```python
from build123d import *

# Parameters (mm, degrees)
DODANIE_WYCI_GNI_CIE1_DEPTH = 5
DODANIE_WYCI_GNI_CIE2_START = 17
SZKIC3_R                    = 12.625
DODANIE_WYCI_GNI_CIE2_DEPTH = 17
SZKIC4_R                    = 2.5
SZKIC4_R_2                  = 1.55
WYTNIJ_WYCI_GNI_CIE1_DEPTH  = 25
SZKIC5_R                    = 3.75
WYTNIJ_WYCI_GNI_CIE2_DEPTH  = 7.5
DODANIE_WYCI_GNI_CIE3_DEPTH = 15
SZKIC7_R                    = 1.5
WYTNIJ_WYCI_GNI_CIE3_DEPTH  = 14
SZKIC8_R                    = 7.5
WYTNIJ_WYCI_GNI_CIE4_DEPTH  = 14
SZKIC14_R                   = 12.625
SZKIC16_R                   = 10.3
SZKIC18_R                   = 3.75
WYTNIJ_WYCI_GNI_CIE5_DEPTH  = 7.5
SZKIC19_R                   = 0.7
WYTNIJ_WYCI_GNI_CIE6_DEPTH  = 5


with BuildPart() as part:
    # Szkic1 → Dodanie-wyciągnięcie1 (new body)
    with BuildSketch(Plane(origin=(0, 0, 0), x_dir=(1, 0, 0), z_dir=(0, 1, 0))):
        with BuildLine():
            Line((-9, 0), (-9, 55.600537222))
            ThreePointArc((-9, 55.600537222), (7.148204378, 68.984355181), (13.393573335, 48.962206087))
            add(Edge.make_bspline(
                [(0, 21.46), (3.478909601, 36.621824573), (13.393573335, 48.962206087)],
                knots=[0, 0, 0, 1, 1, 1], degree=2))
            Line((0, 21.46), (0, 16.16))
            add(Edge.make_bspline(
                [(0, 16.16), (0.310809708, 10.646673881), (5.027347184, 7.464970214)],
                knots=[0, 0, 0, 1, 1, 1], degree=2))
            ThreePointArc((5.027347184, 7.464970214), (4.228112779, -7.945002349), (-9, 0))
        make_face()
    extrude(amount=DODANIE_WYCI_GNI_CIE1_DEPTH)

    # Szkic3 → Dodanie-wyciągnięcie2 (add)
    with BuildSketch(Plane.XZ.offset(DODANIE_WYCI_GNI_CIE2_START)):
        with Locations(Location((3.56, -56.88, 0), (0, 0, 270))):
            Circle(SZKIC3_R)
    extrude(amount=-DODANIE_WYCI_GNI_CIE2_DEPTH)

    # Szkic4 → Wytnij-wyciągnięcie1 (cut)
    with BuildSketch(Plane.XZ.offset(17)):
        with Locations(Location((3.56, -56.88, 0), (0, 0, 270))):
            Circle(SZKIC4_R)
        with Locations(Location((-3.35, -49.97, 0), (0, 0, 270))):
            Circle(SZKIC4_R_2)
        with Locations(Location((10.47, -49.97, 0), (0, 0, 270))):
            Circle(SZKIC4_R_2)
        with Locations(Location((-3.35, -63.79, 0), (0, 0, 270))):
            Circle(SZKIC4_R_2)
        with Locations(Location((10.47, -63.79, 0), (0, 0, 270))):
            Circle(SZKIC4_R_2)
    extrude(amount=-WYTNIJ_WYCI_GNI_CIE1_DEPTH, mode=Mode.SUBTRACT)

    # Szkic5 → Wytnij-wyciągnięcie2 (cut)
    with BuildSketch(Plane.XZ.offset(17)):
        with Locations(Location((3.56, -56.88, 0), (0, 0, 270))):
            Circle(SZKIC5_R)
    extrude(amount=-WYTNIJ_WYCI_GNI_CIE2_DEPTH, mode=Mode.SUBTRACT)

    # Szkic6 → Dodanie-wyciągnięcie3 (add)
    with BuildSketch(Plane(origin=(0, 5, 0), x_dir=(1, 0, 0), z_dir=(0, 1, 0))):
        with BuildLine():
            Line((-9, 55.600537222), (-9, 62.310537222))
            Line((-9, 62.310537222), (-4.379377966, 68.310537222))
            Line((-4.379377966, 68.310537222), (1.560622034, 69.345677388))
            add(Edge.make_bspline(
                [(1.560622034, 69.345677388), (-7.284103586, 65.531370102), (-9, 55.600537222)],
                knots=[0, 0, 0, 1, 1, 1], degree=2))
        make_face()
    extrude(amount=-DODANIE_WYCI_GNI_CIE3_DEPTH)

    # Szkic7 → Wytnij-wyciągnięcie3 (cut)
    with BuildSketch(Plane(origin=(-35.771148282, 0, -27.547492656), x_dir=(-0.6101451639012687, 0, 0.7922896433551899), z_dir=(-0.7922896433551899, 0, -0.6101451639012687))):
        with Locations((-47.663180862, 2)):
            Circle(SZKIC7_R)
        with Locations((-47.663180862, -7)):
            Circle(SZKIC7_R)
    extrude(amount=-WYTNIJ_WYCI_GNI_CIE3_DEPTH, mode=Mode.SUBTRACT)

    # Szkic8 → Wytnij-wyciągnięcie4 (cut)
    with BuildSketch(Plane(origin=(0, 5, 0), x_dir=(1, 0, 0), z_dir=(0, 1, 0))):
        with Locations(Location((0, 0, 0), (0, 0, 270))):
            Circle(SZKIC8_R)
    extrude(amount=-WYTNIJ_WYCI_GNI_CIE4_DEPTH, mode=Mode.SUBTRACT)

    # Szkic14 → Wyciągnięcie po profilach3 section 0
    with BuildSketch(Plane.XZ.offset(17)):
        with Locations((3.56, -56.88)):
            Circle(SZKIC14_R)
    # Szkic16 → Wyciągnięcie po profilach3 section 1
    with BuildSketch(Plane(origin=(0, -26.05, 0), x_dir=(-1, 0, 0), z_dir=(0, -1, 0))):
        with Locations((-3.56, 56.88)):
            Circle(SZKIC16_R)
    loft()

    # Szkic18 → Wytnij-wyciągnięcie5 (cut)
    with BuildSketch(Plane.XZ.offset(26.05)):
        with Locations(Location((3.56, -56.88, 0), (0, 0, 270))):
            Circle(SZKIC18_R)
    extrude(amount=-WYTNIJ_WYCI_GNI_CIE5_DEPTH, mode=Mode.SUBTRACT)

    # Szkic19 → Wytnij-wyciągnięcie6 (cut)
    with BuildSketch(Plane.XZ.offset(26.05)):
        with Locations(Location((-3.68, -53.48, 0), (0, 0, 270))):
            Circle(SZKIC19_R)
        with Locations(Location((-3.68, -56.88, 0), (0, 0, 270))):
            Circle(SZKIC19_R)
        with Locations(Location((-3.68, -60.28, 0), (0, 0, 270))):
            Circle(SZKIC19_R)
        with Locations(Location((0.16, -64.12, 0), (0, 0, 270))):
            Circle(SZKIC19_R)
        with Locations(Location((3.56, -64.12, 0), (0, 0, 270))):
            Circle(SZKIC19_R)
        with Locations(Location((6.96, -64.12, 0), (0, 0, 270))):
            Circle(SZKIC19_R)
        with Locations(Location((10.8, -60.28, 0), (0, 0, 270))):
            Circle(SZKIC19_R)
        with Locations(Location((10.8, -56.88, 0), (0, 0, 270))):
            Circle(SZKIC19_R)
        with Locations(Location((10.8, -53.639400789, 0), (0, 0, 270))):
            Circle(SZKIC19_R)
        with Locations(Location((6.96, -49.64, 0), (0, 0, 270))):
            Circle(SZKIC19_R)
        with Locations(Location((3.56, -49.64, 0), (0, 0, 270))):
            Circle(SZKIC19_R)
        with Locations(Location((0.16, -49.64, 0), (0, 0, 270))):
            Circle(SZKIC19_R)
    extrude(amount=-WYTNIJ_WYCI_GNI_CIE6_DEPTH, mode=Mode.SUBTRACT)


solid = part.part
```
Verification items for the finished model (mm, model axes). A direction names the side the tool comes from. Coordinates: 2 decimals unless noted, no trailing zeros. Order: outer loops, then holes, each group sorted by start corner. A loop starts at its lowest first (then second) coordinate and runs counter-clockwise, first axis right, second up. Notation, with made-up numbers: (73.25, -22) -> (130.25, -22) arc R31 ccw to (130.25, 2) -> close; hole circle Ø11 at (70, -9.5). An arc over 180 degrees is marked (long way). Put each result on its own line as item: value. Start each with the question number.
1) Material ranges on L1, parallel to X at y = -24, z = -60; L2, parallel to X at y = -3.25, z = -56.88 (3 decimals); L3, parallel to X at y = -7, z = -63, recorded low to high.
2) Go/stop test with flat-tipped pins: pin 1 (1.2 mm diameter, centred on y = -4, z = -59.5, fed in from -X); pin 2 (2 mm diameter, centred on x = 7, y = -20.5, fed in from -Z); pin 3 (6 mm diameter, centred on x = 3, y = -1.5, fed in from +Z). Record where each tip stops, or that it passes through.
3) Cross-section at A-A (z = -5.5). Enter the section's corners in (x, y).
4) Cross-section at B-B (y = -20). Enter the section's corners in (x, z), plus the area to 3 significant figures.
5) Tool access check on faces 1 (the cylindrical face through (10.83, -23.58, -59.58)), 2 (the flat face through (-6.1, -10, -65.4)), 3 (the flat face through (1, -9.5, -58)), 4 (the flat face through (10, -17, -50)). Record the directions out of +Z, -Z, +X, -X, +Y, -Y that give a thin tool (end or side, any length) a straight path to the whole face; none if there is none.
6) Cross-section at C-C (z = -20). Enter the section's corners in (x, y), plus the area to 3 significant figures.
7) Release check for a two-part mould opening along Y. For faces 5 (the flat face through (-3, 0, -24)), 6 (the cylindrical face through (3.725, -13.302, -53.134)), 7 (the cylindrical face through (10.54, -6.15, -48.42)), 8 (the cylindrical face through (-3.004, -6.549, -60.667)) record: pulls with the +Y half, pulls with the -Y half, needs draft (parallel to the pull), parting line crosses it, or undercut.
Geometry check:
1. L1: x = -6.81 to -4.32, -3.04 to 1.48, 5.64 to 10.16, 11.44 to 13.93
1. L2: x = -9.065 to 1.06, 6.06 to 16.185
1. L3: x = -8.47 to -6.15, -1.23 to 9.14, 11.8 to 14.6
2. pin 1: stops at x = -9
2. pin 2: stops at z = -68.47
2. pin 3: stops at z = 8.99
3. outline: (-9, 0) -> (-5.1, 0) -> (-5.1, 5) -> (-9, 5) -> close; (5.1, 0) -> (7.12, 0) -> (7.12, 5) -> (5.1, 5) -> close
4. outline: circle Ø23.71 at (3.56, -56.88); hole circle Ø7.5 at (3.56, -56.88)
4. area: 397 mm^2
5. face 1: -Y
5. face 2: -Z, -X, -Y
5. face 3: none
5. face 4: +Y
6. outline: (-9, 0) -> (0, 0) -> (0, 5) -> (-9, 5) -> close
6. area: 45.0 mm^2
7. face 5: pulls with the -Y half
7. face 6: undercut
7. face 7: needs draft
7. face 8: undercut
